from build123d import *

# Parameters (mm, degrees)
SKETCH1_R           = 1.5
BOSS_EXTRUDE1_DEPTH = 3
FILLET1_R           = 6
FILLET2_R           = 3
CUT_EXTRUDE1_REACH  = 5
SKETCH2_R           = 1.5


with BuildPart() as part:
    # Sketch1 → Boss-Extrude1 (new body)
    with BuildSketch(Plane(origin=(0, 0, 0), x_dir=(1, 0, 0), z_dir=(0, 1, 0))):
        with BuildLine():
            Line((-74.629040009, 40.687914512), (-63.639610307, 29.69848481))
            Line((-63.639610307, 29.69848481), (-42.426406871, 50.911688245))
            Line((-42.426406871, 50.911688245), (-36.769552622, 45.254833996))
            Line((-36.769552622, 45.254833996), (-68.72500623, 13.299380388))
            ThreePointArc((-68.72500623, 13.299380388), (-69.616532676, 7.316992429), (-69.988296617, 1.279975229))
            Line((-69.988296617, 1.279975229), (-45.375058731, -36.621087439))
            Line((-45.375058731, -36.621087439), (-52.084423274, -40.978199719))
            Line((-52.084423274, -40.978199719), (-68.423594325, -15.81808268))
            Line((-68.423594325, -15.81808268), (-81.457709532, -24.282536066))
            ThreePointArc((-81.457709532, -24.282536066), (-84.534361106, 8.884919378), (-74.629040009, 40.687914512))
        make_face()
        with Locations((-43.840620434, 43.840620434)):
            Circle(SKETCH1_R, mode=Mode.SUBTRACT)
        with Locations((-59.39696962, 28.284271247)):
            Circle(SKETCH1_R, mode=Mode.SUBTRACT)
        with Locations((-51.997575213, -33.767620171)):
            Circle(SKETCH1_R, mode=Mode.SUBTRACT)
        with Locations((-63.979633983, -15.316867676)):
            Circle(SKETCH1_R, mode=Mode.SUBTRACT)
    extrude(amount=BOSS_EXTRUDE1_DEPTH)

    # Fillet1
    fillet1_edges = [part.edges().sort_by_distance(p)[0] for p in [
        (-74.629040009, 1.5, -40.687914512),
        (-81.457709532, 1.5, 24.282536066),
    ]]
    fillet(fillet1_edges, radius=FILLET1_R)

    # Fillet2
    fillet2_edges = [part.edges().sort_by_distance(p)[0] for p in [
        (-63.639610307, 1.5, -29.69848481),
        (-68.72500623, 1.5, -13.299380388),
        (-69.988296617, 1.5, -1.279975229),
        (-68.423594325, 1.5, 15.81808268),
    ]]
    fillet(fillet2_edges, radius=FILLET2_R)

    # Sketch2 → Cut-Extrude1 (cut, up to next)
    with BuildSketch(Plane(origin=(0, 3, 0), x_dir=(1, 0, 0), z_dir=(0, 1, 0)), mode=Mode.PRIVATE) as cut_extrude1_sk1:
        with Locations((-79.5, 8.5)):
            Circle(SKETCH2_R)
    cut_extrude1_tool1 = extrude(cut_extrude1_sk1.sketch, amount=-CUT_EXTRUDE1_REACH, mode=Mode.PRIVATE) & part.part
    add(cut_extrude1_tool1.solids().sort_by_distance((-79.5, 3, -8.5))[0], mode=Mode.SUBTRACT)


solid = part.part
For this review, take the finished solid that the model builds, in its own axes (mm). A direction names the side the tool comes from. Give positions to 0.01 mm unless a question says otherwise; leave off trailing zeros. Loops run counter-clockwise (first coordinate to the right, second up) from the corner with the lowest first, then second, coordinate; pieces in that order, holes last.
Item 1: Take a section at C-C, the plane y = 0.8. State the section outline as (x, z) points, and give its area (3 significant figures).
Item 2: Insertion check: pin 1 (1.5 mm diameter, centred on x = -56.5, y = 1, fed in from -Z). The pin has a flat end and moves straight along its axis. Give the tip position at first contact, or say it passes through.
Item 3: Tool access review of faces 4 (the cylindrical face through (-58.705, 1.479, -26.954)), 5 (the flat face through (-52.2, 1.479, -29.825)), 6 (the flat face through (-72.63, 1.48, 18.55)): name each direction out of +Z, -Z, +X, -X, +Y, -Y from which nothing blocks a thin tool from reaching the whole face with its end or side.
Item 4: Take a section at A-A, the plane x = -60. State the section outline as (y, z) points, and give its area (3 significant figures).
Item 5: For line 1 along Z through (x, y) = (-60, 1.3); line 2 along Z through (x, y) = (-59, 1.75); line 3 along Z through (x, y) = (-45.5, 2.3), list the stretches that pass through material, from the lowest coordinate up.
Item 6: Draft analysis for pull direction X (two halves, no side actions). For faces 1 (the cylindrical face through (-84.57, 1.48, -8.54)), 2 (the flat face through (-52.11, 1.48, -41.23)), 3 (the flat face through (-48.683, 1.479, 38.769)), state which applies: +X half, -X half, draft (parallel to the pull), parting line (faces both ways), or undercut.
Item 7: Take a section at D-D, the plane x = -46.5. State the section outline as (y, z) points, and give its area (3 significant figures).
Item 8: Take a section at B-B, the plane z = -8.5. State the section outline as (x, y) points, and give its area (3 significant figures).
Calculated:
1. outline: (-83.53, 15.76) arc R85 ccw to (-78.43, -32.78) arc R6 ccw to (-68.65, -34.71) - (-65.76, -31.82) arc R3 cw to (-61.52, -31.82) - (-42.43, -50.91) - (-36.77, -45.25) - (-68.07, -13.96) arc R3 cw to (-68.9, -12.37) arc R70 cw to (-69.96, -2.23) arc R3 cw to (-69.48, -0.5) - (-45.38, 36.62) - (-52.08, 40.98) - (-66.79, 18.33) arc R3 cw to (-70.94, 17.45) - (-74.36, 19.68) arc R6 ccw to start; hole circle Ø3 at (-79.5, -8.5); hole circle Ø3 at (-63.98, 15.32); hole circle Ø3 at (-59.4, -28.28); hole circle Ø3 at (-52, 33.77); hole circle Ø3 at (-43.84, -43.84)
1. area: 1,390 mm2
2. pin 1: stops at z = -37.59
3. face 4: +Y, -Y
3. face 5: +X, +Y, -Y
3. face 6: +Z, +Y, -Y
4. outline: (0, -33.34) - (3, -33.34) - (3, -29.66) - (0, -29.66) - close; (0, -26.91) - (3, -26.91) - (3, -22.02) - (0, -22.02) - close; (0, 14.1) - (3, 14.1) - (3, 28.79) - (0, 28.79) - close
4. area: 69.8 mm2
5. line 1: z = -33.34 to -29.66, -26.91 to -22.02, 14.1 to 28.79
5. line 2: z = -34.34 to -29.73, -26.84 to -23.02, 15.64 to 30.33
5. line 3: z = -47.84 to -36.52, 36.43 to 36.7
6. face 1: -X half
6. face 2: undercut
6. face 3: +X half
7. outline: (0, -46.84) - (3, -46.84) - (3, -35.52) - (0, -35.52) - close; (0, 34.89) - (3, 34.89) - (3, 37.35) - (0, 37.35) - close
7. area: 41.3 mm2
8. outline: (-84.57, 0) - (-81, 0) - (-81, 3) - (-84.57, 3) - close; (-78, 0) - (-69.48, 0) - (-69.48, 3) - (-78, 3) - close
8. area: 36.3 mm2
